Can you work these out from the model? Positions are in its coordinate system, mm. A direction names the side the tool comes from. Round coordinates to 2 decimals unless told otherwise and drop trailing zeros. Loops run counter-clockwise (first coordinate to the right, second up) from the corner with the lowest first, then second, coordinate; pieces in that order, holes last. Notation, with made-up numbers: (-31.75, 46) - (0.25, 46) arc R37 ccw to (0.25, 85) - close; hole circle Ø5 at (65.25, -28). An arc over 180 degrees is marked (long way). Answer as CSV lines item,"result".
Autodesk Inventor part; units mm, degrees
ref_plane "YZ Plane" through (0, 0, 0) normal (1, 0, 0) x (0, 1, 0)
ref_plane "XY Plane" through (0, 0, 0) normal (0, 0, 1) x (1, 0, 0)
sketch "Skizze1" plane through (0, 0, 0) normal (0, 0, 1) x (1, 0, 0)
  line L0 (0, 0) -> (5, 0)
  line L1 (5, 0) -> (5, 8)
  line L2 (5, 8) -> (4, 8)
  line L3 (4, 8) -> (4, 1)
  line L4 (4, 1) -> (0, 1)
  line L5 (0, 9.6) -> (0, -1.6) construction
  line L6 (0, 0) -> (-5, 0)
  line L7 (-5, 0) -> (-5, 8)
  line L8 (-5, 8) -> (-4, 8)
  line L9 (-4, 8) -> (-4, 1)
  line L10 (-4, 1) -> (0, 1)
  dimension "d0" = 1
  dimension "d1" = 1
  dimension "d2" = 8
  dimension "d3" = 5
extrude "Ex-UProfil" add sketch "Skizze1" along normal blind 265
sketch "Skizze2" plane through (0, 0, 0) normal (0, 1, 0) x (-1, 0, 0)
  line L0 (5, 0) -> (-5, 0)
  line L1 (-5, 0) -> (-5, 265)
  line L2 (5, 265) -> (-5, 265)
  line L3 (5, 0) -> (5, 265)
  line L4 (0, -65.78) -> (0, 302.63) construction
  circle A0 centre (0, 245) radius 2.15 construction
  line L5 (0, 246) -> (0, 244) construction
  line L6 (-2.15, 246) -> (-2.15, 244)
  line L7 (2.15, 244) -> (2.15, 246)
  arc A1 (2.15, 246) -> (-2.15, 246) centre (0, 246) ccw
  arc A2 (-2.15, 244) -> (2.15, 244) centre (0, 244) ccw
  circle A3 centre (0, 165) radius 2.15 construction
  line L8 (0, 166) -> (0, 164) construction
  line L9 (-2.15, 166) -> (-2.15, 164)
  line L10 (2.15, 164) -> (2.15, 166)
  arc A4 (2.15, 166) -> (-2.15, 166) centre (0, 166) ccw
  arc A5 (-2.15, 164) -> (2.15, 164) centre (0, 164) ccw
  circle A6 centre (0, 85) radius 2.15 construction
  line L11 (0, 86) -> (0, 84) construction
  line L12 (-2.15, 86) -> (-2.15, 84)
  line L13 (2.15, 84) -> (2.15, 86)
  arc A7 (2.15, 86) -> (-2.15, 86) centre (0, 86) ccw
  arc A8 (-2.15, 84) -> (2.15, 84) centre (0, 84) ccw
  circle A9 centre (0, 5) radius 2.15 construction
  line L14 (0, 6) -> (0, 4) construction
  line L15 (-2.15, 6) -> (-2.15, 4)
  line L16 (2.15, 4) -> (2.15, 6)
  arc A10 (2.15, 6) -> (-2.15, 6) centre (0, 6) ccw
  arc A11 (-2.15, 4) -> (2.15, 4) centre (0, 4) ccw
  point P0 (0, 0)
  point P1 (0, 248.15)
  point P2 (0, 241.85)
  point P3 (0, 168.15)
  point P4 (0, 161.85)
  point P5 (0, 88.15)
  point P6 (0, 81.85)
  point P7 (0, 8.15)
  point P8 (0, 1.85)
  dimension "d6" = 4.3
  dimension "d7" = 20
  dimension "d8" = 4.3
  dimension "d9" = 6.3
  dimension "d21" = 80
extrude "Ex-Bohrungen" cut sketch "Skizze2" along normal up to surface (1 mm away) contours A1 L7 A2 L6 | A4 L10 A5 L9 | A7 L13 A8 L12 | A10 L16 A11 L15
equation "\"d8\" = d6"
properties part number "U-Profil PanelSupport 10x8x265mm"
Q1. On a 3-axis mill with a long thin cutter (end or side, diameter ignored), from which of +Z, -Z, +X, -X, +Y, -Y can I reach the whole of each face in a straight line? I mean faces 1 (the flat face through (4, 5, 131)), 2 (the flat face through (0, 0.8, 265)). Say none if no direction works.
Checks:
face 1,"+Z, -Z, +Y"
face 2,"+Z, +X, -X, +Y, -Y"
Q2. Imagine slicing it at B-B (y = 2.5). Write out the boundary of the cut face in (x, z), then the cut area to 3 significant figures.
Checks:
outline,"(-5, 0) - (-4, 0) - (-4, 265) - (-5, 265) - close; (4, 0) - (5, 0) - (5, 265) - (4, 265) - close"
area,"530 mm²"
Q3. We'd pull the mould along X, two halves only. Please class faces 3 (the flat face through (-4, 5, 131)), 4 (the flat face through (-5, 4, 131)), 5 (the flat face through (5, 4, 131)): pulls with the +X half, pulls with the -X half, needs draft (parallel to the pull), parting line crosses it, or undercut.
Checks:
face 3,"undercut"
face 4,"pulls with the -X half"
face 5,"pulls with the +X half"
Q4. If I drill on line 1 along X through (y, z) = (3, 66); line 2 along Z through (x, y) = (-1.25, 0.5); line 3 along Y through (x, z) = (-3.25, 115), over which ranges is the centre line in solid material (lowest first)? Write a range as [from, to].
Checks:
line 1,"[-5, -4], [4, 5]"
line 2,"[0, 2.25], [7.75, 82.25], [87.75, 162.25], [167.75, 242.25], [247.75, 265]"
line 3,"[0, 1]"
Q5. Imagine slicing it at C-C (z = 77.5). Write out the boundary of the cut face in (x, y).
Checks:
outline,"(-5, 0) - (5, 0) - (5, 8) - (4, 8) - (4, 1) - (-4, 1) - (-4, 8) - (-5, 8) - close"
Q6. I'm going to push flat-ended pins straight in: pin 1 Ø1 at (x, z) = (1.5, 205.5) entering from +Y; pin 2 Ø1 at (x, y) = (-2, 2.5) entering from +Z. Where does each tip first touch, or does it pass through?
Checks:
pin 1,"y = 1"
pin 2,"through"
Q7. Imagine slicing it at A-A (x = 0). Write out the boundary of the cut face in (y, z).
Checks:
outline,"(0, 0) - (1, 0) - (1, 1.85) - (0, 1.85) - close; (0, 8.15) - (1, 8.15) - (1, 81.85) - (0, 81.85) - close; (0, 88.15) - (1, 88.15) - (1, 161.85) - (0, 161.85) - close; (0, 168.15) - (1, 168.15) - (1, 241.85) - (0, 241.85) - close; (0, 248.15) - (1, 248.15) - (1, 265) - (0, 265) - close"
